Design review of the part shown in the three views and the two pictorial views. Dimensions are in mm from the part's minimum x, y and z. A direction names the side the tool comes from. Give positions to 0.01 mm unless a question says otherwise; leave off trailing zeros. Loops run counter-clockwise (first coordinate to the right, second up) from the corner with the lowest first, then second, coordinate; pieces in that order, holes last. Notation, with made-up numbers: (41.5, 28.5) -> (84.5, 28.5) arc R33 ccw to (84.5, 63.5) -> close; hole circle Ø6 at (20, 87). An arc over 180 degrees is marked (long way). Use CSV: the item, a comma, the result in double quotes. Start each with the question number.
Item 1: We need section D-D (y = 14). State the section outline as (x, z) points.
Item 2: We need section A-A (y = 11). State the section outline as (x, z) points, plus the area to 3 significant figures.
Item 3: The part is to be moulded in two halves that separate along Y. For the marked faces 3, 4, 5 and 6, say which applies: +Y half, -Y half, draft (parallel to the pull), parting line (faces both ways), or undercut.
Item 4: For the marked faces 1 and 2, list the 3-axis set-ups (+Z, -Z, +X, -X, +Y, -Y) from which the entire face can be reached by the end or side of a thin tool; tool diameter is ignored.
Item 5: Wall thickness on line 1 along Y through (x, z) = (6, 0.85); line 2 along Y through (x, z) = (1.35, 11); line 3 along X through (y, z) = (10.25, 13.25): over which ranges is each line inside the solid? List them lowest first. Write a range as from..to.
Item 6: We need section C-C (x = 5.25). State the section outline as (y, z) points.
Item 7: Clearance check with flat-ended pins moving along their axes: pin 1 (6 mm diameter, centred on x = 5.5, y = 12, fed in from -Z); pin 2 (6.5 mm diameter, centred on y = 5, z = 7, fed in from +X); pin 3 (2.5 mm diameter, centred on x = 6.5, y = 9.5, fed in from +Z). State where each tip first meets the part, or that it passes through.
Item 8: We need section B-B (z = 11). State the section outline as (x, y) points.
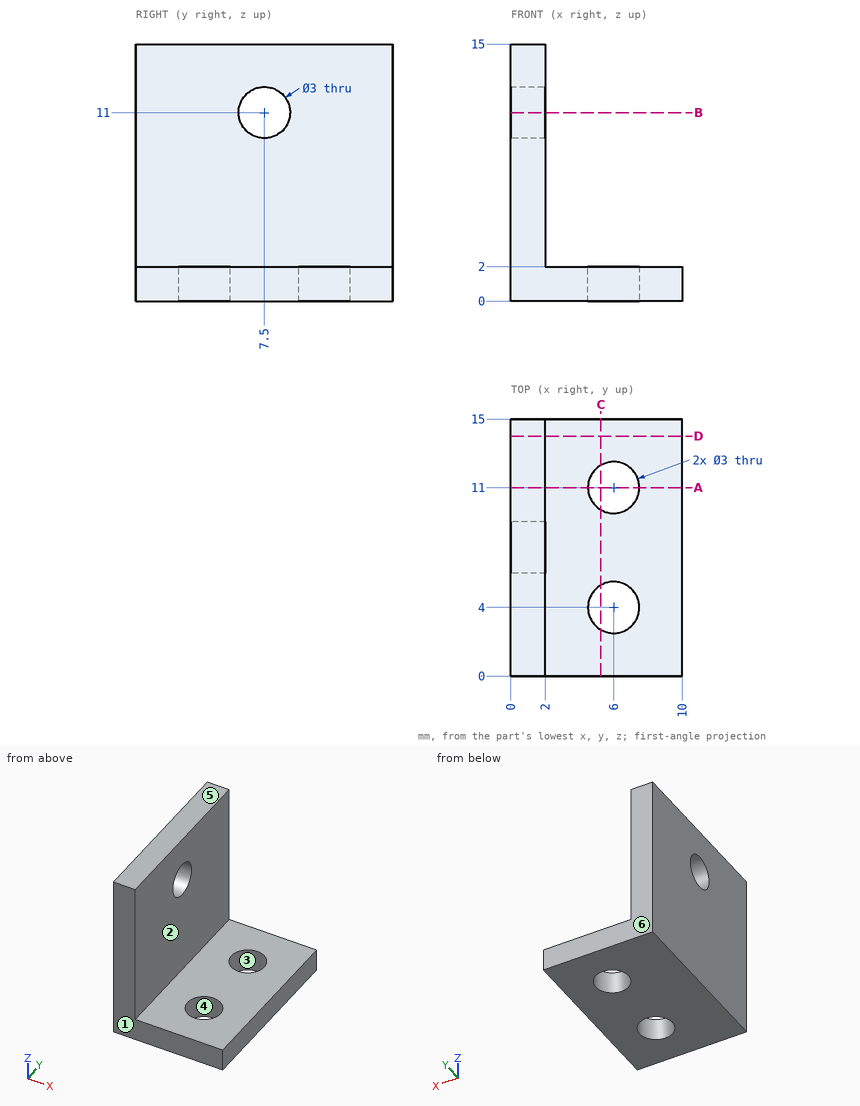
Results found:
1,outline,"(0, 0) -> (10, 0) -> (10, 2) -> (2, 2) -> (2, 15) -> (0, 15) -> close"
2,outline,"(0, 0) -> (4.5, 0) -> (4.5, 2) -> (2, 2) -> (2, 15) -> (0, 15) -> close; (7.5, 0) -> (10, 0) -> (10, 2) -> (7.5, 2) -> close"
2,area,"40.0 mm²"
3,face 3,"undercut"
3,face 4,"undercut"
3,face 5,"draft"
3,face 6,"+Y half"
4,face 1,"+Z, -Z, +X, -X, -Y"
4,face 2,"+Z, +X, +Y, -Y"
5,line 1,"0..2.5, 5.5..9.5, 12.5..15"
5,line 2,"0..6, 9..15"
5,line 3,"0..2"
6,outline,"(0, 0) -> (2.7, 0) -> (2.7, 2) -> (0, 2) -> close; (5.3, 0) -> (9.7, 0) -> (9.7, 2) -> (5.3, 2) -> close; (12.3, 0) -> (15, 0) -> (15, 2) -> (12.3, 2) -> close"
7,pin 1,"z = 0"
7,pin 2,"x = 2"
7,pin 3,"z = 2"
8,outline,"(0, 0) -> (2, 0) -> (2, 6) -> (0, 6) -> close; (0, 9) -> (2, 9) -> (2, 15) -> (0, 15) -> close"
